Can you work these out from the model? Positions are in its coordinate system, mm. Give positions to 0.01 mm unless a question says otherwise; leave off trailing zeros. Order: outer loops, then holes, each group sorted by start corner. A loop starts at its lowest first (then second) coordinate and runs counter-clockwise, first axis right, second up. Notation, with made-up numbers: (33.25, 2.5) - (74.25, 2.5) arc R5 cw to (74.25, 9.5) - close; hole circle Ø5 at (70.25, -33.75). An arc over 180 degrees is marked (long way). One line per question, with ' | ' between items.
```python
from build123d import *

# Parameters (mm, degrees)
BOSS_EXTRUDE1_DEPTH = 0.375


with BuildPart() as part:
    # Sketch3 → Boss-Extrude1 (new, symmetric)
    with BuildSketch(Plane.XY):
        with BuildLine():
            Line((-2.800142094, -5.780594647), (-2.800142094, -4.16896088))
            ThreePointArc((-2.800142094, -4.16896088), (-2.906194065, -3.675728978), (-3.205604942, -3.269677435))
            ThreePointArc((-3.205604942, -3.269677435), (-4.528005601, 2.072292656), (0, 5.2))
            Line((0, 5.2), (0, 3.7))
            ThreePointArc((0, 3.7), (-3.69774606, 0.129128138), (-0.258098953, -3.690986986))
            Line((-0.258098953, -3.690986986), (-0.409154928, -4.520936126))
            Line((-0.409154928, -4.520936126), (-1.019085782, -4.552901247))
            ThreePointArc((-1.019085782, -4.552901247), (-1.586861929, -5.120677394), (-1.081544887, -5.744691972))
            Line((-1.081544887, -5.744691972), (-0.746581142, -5.797745018))
            ThreePointArc((-0.746581142, -5.797745018), (-0.504992542, -5.933041134), (-0.409154928, -6.192820354))
            Line((-0.409154928, -6.192820354), (-0.409154928, -6.870700795))
            ThreePointArc((-0.409154928, -6.870700795), (-0.419264451, -6.894041896), (-0.443205367, -6.902635035))
            ThreePointArc((-0.443205367, -6.902635035), (-1.364795043, -6.780865425), (-2.261733258, -6.536617175))
            ThreePointArc((-2.261733258, -6.536617175), (-2.651783457, -6.244667416), (-2.800142094, -5.780594647))
        make_face()
    extrude(amount=BOSS_EXTRUDE1_DEPTH, both=True)

    # Mirror1: part across plane


with BuildPart() as part_1:
    add(part.part)
    add(part.part.mirror(Plane(origin=(0, 5.2, 0.375), x_dir=(0, 0, 1), z_dir=(-1, 0, 0))))


solid = part_1.part
```
(1) If I drill on line 1 (Y direction, x = -0.5, z = -0.25); line 2 (Y direction, x = -1.25, z = -0.2); line 3 (X direction, y = -0.75, z = 0.2), over which ranges is the centre line in solid material (lowest first)?
Answer below:
line 1: -6.9 to -5.94, -4.53 to -3.67, 3.67 to 5.17 | line 2: -6.8 to -5.69, -4.61 to -3.48, 3.48 to 5.04 | line 3: -4.71 to -3.62, 3.62 to 4.71
(2) Imagine slicing it at B-B (z = -0.1). List the corners of the cut face in (x, y) for me.
Answer below:
outline: (-3.21, -3.27) arc R1.2 cw to (-2.8, -4.17) - (-2.8, -5.78) arc R0.8 ccw to (-2.26, -6.54) arc R6.92 ccw to (-0.44, -6.9) arc R0.03 ccw to (-0.41, -6.87) - (-0.41, -6.19) arc R0.4 ccw to (-0.75, -5.8) - (-1.08, -5.74) arc R0.6 cw to (-1.02, -4.55) - (-0.41, -4.52) - (-0.26, -3.69) arc R3.7 cw (long way) to (0.26, -3.69) - (0.41, -4.52) - (1.02, -4.55) arc R0.6 cw to (1.08, -5.74) - (0.75, -5.8) arc R0.4 ccw to (0.41, -6.19) - (0.41, -6.87) arc R0.03 ccw to (0.44, -6.9) arc R6.92 ccw to (2.26, -6.54) arc R0.8 ccw to (2.8, -5.78) - (2.8, -4.17) arc R1.2 cw to (3.21, -3.27) arc R4.84 ccw (long way) to start
(3) Imagine slicing it at D-D (y = 4). List the corners of the cut face in (x, z) for me (3 decimals).
Answer below:
outline: (-3.191, -0.375) - (3.191, -0.375) - (3.191, 0.375) - (-3.191, 0.375) - close
(4) If we mould it in two halves opening along Z, with no side actions, what happens to faces 1 (the face through (-4, -1, 0.375)), 2 (the face through (-4, -1, -0.375))? For each: released by +Z, released by -Z, zero draft, split by the parting line, or undercut.
Answer below:
face 1: released by +Z | face 2: released by -Z
(5) Imagine slicing it at C-C (x = 3). List the corners of the cut face in (y, z) for me (1 decimal).
Answer below:
outline: (-3.5, -0.4) - (-2.2, -0.4) - (-2.2, 0.4) - (-3.5, 0.4) - close; (2.2, -0.4) - (4.2, -0.4) - (4.2, 0.4) - (2.2, 0.4) - close
(6) Will this pin go through, and if not, where does the flat tip stop? pin 1 (3 mm diameter, centred on x = -3.5, y = -4.5, fed in from -Z) (3 decimals).
Answer below:
pin 1: z = -0.375
(7) Imagine slicing it at A-A (y = -1.5). List the corners of the cut face in (x, z) for me (3 decimals).
Answer below:
outline: (-4.471, -0.375) - (-3.382, -0.375) - (-3.382, 0.375) - (-4.471, 0.375) - close; (3.382, -0.375) - (4.471, -0.375) - (4.471, 0.375) - (3.382, 0.375) - close
